from build123d import *

# Parameters (mm, degrees)
BASE_FLANGE1_DEPTH = 27
SKETCH2_R          = 3
CUT_EXTRUDE1_DEPTH = 10
CHAMFER1_SIZE      = 2


# Sheet-metal steps are written as plain solids
with BuildPart() as part:
    # Sketch1 → Base-Flange1 (new, symmetric)
    with BuildSketch(Plane.XY):
        with BuildLine():
            Line((95, -32.5), (81, -32.5))
            ThreePointArc((81, -32.5), (78.878679656, -31.621320344), (78, -29.5))
            Line((78, -29.5), (78, 31))
            ThreePointArc((78, 31), (77.560660172, 32.060660172), (76.5, 32.5))
            Line((76.5, 32.5), (-76.5, 32.5))
            ThreePointArc((-76.5, 32.5), (-77.560660172, 32.060660172), (-78, 31))
            Line((-78, 31), (-78, -29.5))
            ThreePointArc((-78, -29.5), (-78.878679656, -31.621320344), (-81, -32.5))
            Line((-81, -32.5), (-95, -32.5))
            Line((-95, -32.5), (-95, -31))
            Line((-95, -31), (-81, -31))
            ThreePointArc((-81, -31), (-79.939339828, -30.560660172), (-79.5, -29.5))
            Line((-79.5, -29.5), (-79.5, 31))
            ThreePointArc((-79.5, 31), (-78.621320344, 33.121320344), (-76.5, 34))
            Line((-76.5, 34), (76.5, 34))
            ThreePointArc((76.5, 34), (78.621320344, 33.121320344), (79.5, 31))
            Line((79.5, 31), (79.5, -29.5))
            ThreePointArc((79.5, -29.5), (79.939339828, -30.560660172), (81, -31))
            Line((81, -31), (95, -31))
            Line((95, -31), (95, -32.5))
        make_face()
    extrude(amount=BASE_FLANGE1_DEPTH, both=True)

    # Sketch2 → Cut-Extrude1 (cut)
    with BuildSketch(Plane(origin=(0, -31, 0), x_dir=(1, 0, 0), z_dir=(0, 1, 0))):
        with Locations(Location((-87.5, -15, 0), (0, 0, 270))):
            Circle(SKETCH2_R)
        with Locations(Location((87.5, -15, 0), (0, 0, 90))):
            Circle(SKETCH2_R)
        with Locations(Location((87.5, 15, 0), (0, 0, 270))):
            Circle(SKETCH2_R)
        with Locations(Location((-87.5, 15, 0), (0, 0, 90))):
            Circle(SKETCH2_R)
    extrude(amount=-CUT_EXTRUDE1_DEPTH, mode=Mode.SUBTRACT)

    # Chamfer1
    chamfer1_edges = [part.edges().sort_by_distance(p)[0] for p in [
        (95, -31.75, -27),
        (-95, -31.75, -27),
        (95, -31.75, 27),
        (-95, -31.75, 27),
    ]]
    chamfer(chamfer1_edges, length=CHAMFER1_SIZE)


solid = part.part
Input: part model. Units: mm. Frame: model coordinates. A direction names the side the tool comes from. Coordinates: 2 decimals unless noted, no trailing zeros. Order: outer loops, then holes, each group sorted by start corner. A loop starts at its lowest first (then second) coordinate and runs counter-clockwise, first axis right, second up. Notation, with made-up numbers: M 53.5,40.5 L 62.5,40.5 A22 ccw 62.5,47.5 Z; hole C 57.25,-27.5 d7. An arc over 180 degrees is marked long. Answer in a Markdown table with one row per item.
(1) Section query D-D, the plane z = 7. Output: boundary loops of the cut face in (x, y).
Numbers:
| item | result |
|---|---|
| outline | M -95,-32.5 L -81,-32.5 A3 ccw -78,-29.5 L -78,31 A1.5 cw -76.5,32.5 L 76.5,32.5 A1.5 cw 78,31 L 78,-29.5 A3 ccw 81,-32.5 L 95,-32.5 L 95,-31 L 81,-31 A1.5 cw 79.5,-29.5 L 79.5,31 A3 ccw 76.5,34 L -76.5,34 A3 ccw -79.5,31 L -79.5,-29.5 A1.5 cw -81,-31 L -95,-31 Z |
(2) Section query B-B, the plane z = -15. Output: boundary loops of the cut face in (x, y).
Numbers:
| item | result |
|---|---|
| outline | M -95,-32.5 L -90.5,-32.5 L -90.5,-31 L -95,-31 Z; M -84.5,-32.5 L -81,-32.5 A3 ccw -78,-29.5 L -78,31 A1.5 cw -76.5,32.5 L 76.5,32.5 A1.5 cw 78,31 L 78,-29.5 A3 ccw 81,-32.5 L 84.5,-32.5 L 84.5,-31 L 81,-31 A1.5 cw 79.5,-29.5 L 79.5,31 A3 ccw 76.5,34 L -76.5,34 A3 ccw -79.5,31 L -79.5,-29.5 A1.5 cw -81,-31 L -84.5,-31 Z; M 90.5,-32.5 L 95,-32.5 L 95,-31 L 90.5,-31 Z |
(3) Access query for faces 1 (the flat face through (-79.5, 0, 0)), 2 (the flat face through (88, -31, 0)), 3 (the flat face through (-78, 1, 0)). Directions: +Z, -Z, +X, -X, +Y, -Y. A direction counts if a zero-diameter tool reaches every point of the face in a straight line with its end or side. Return the directions, or none.
Numbers:
| item | result |
|---|---|
| face 1 | +Z, -Z, -X, +Y |
| face 2 | +Z, -Z, +X, +Y |
| face 3 | +Z, -Z, -Y |
(4) Section query C-C, the plane x = -87.5. Output: boundary loops of the cut face in (y, z), plus the area to 3 significant figures.
Numbers:
| item | result |
|---|---|
| outline | M -32.5,-27 L -31,-27 L -31,-18 L -32.5,-18 Z; M -32.5,-12 L -31,-12 L -31,12 L -32.5,12 Z; M -32.5,18 L -31,18 L -31,27 L -32.5,27 Z |
| area | 63.0 mm^2 |
(5) Contact query for flat-ended pins moving along their axis: pin 1 Ø6 at (y, z) = (-20.5, -4) entering from -X; pin 2 Ø16 at (y, z) = (-7.5, -5.5) entering from +X; pin 3 Ø5 at (x, z) = (87.5, 15) entering from +Y; pin 4 Ø7 at (x, z) = (90, -7) entering from +Y. Output: stop coordinate, or through.
Numbers:
| item | result |
|---|---|
| pin 1 | stops at x = -79.5 |
| pin 2 | stops at x = 79.5 |
| pin 3 | passes through |
| pin 4 | stops at y = -31 |
(6) Draft query along X for faces 4 (the flat face through (79.5, 1, 0)), 5 (the flat face through (1, 32.5, 0)), 6 (the flat face through (-88, -31, 0)). Return one class per face: pulls with the +X half, pulls with the -X half, needs draft (parallel to the pull), parting line crosses it, or undercut.
Numbers:
| item | result |
|---|---|
| face 4 | pulls with the +X half |
| face 5 | undercut |
| face 6 | needs draft |
(7) Section query A-A, the plane y = -15. Output: boundary loops of the cut face in (x, z), plus the area to 3 significant figures.
Numbers:
| item | result |
|---|---|
| outline | M -79.5,-27 L -78,-27 L -78,27 L -79.5,27 Z; M 78,-27 L 79.5,-27 L 79.5,27 L 78,27 Z |
| area | 162 mm^2 |
(8) Material intervals for line 1 (X direction, y = -1, z = -2); line 2 (X direction, y = -31.55, z = -15); line 3 (X direction, y = -31.8, z = 15), sorted ascending. Write a range as [from, to].
Numbers:
| item | result |
|---|---|
| line 1 | x = [-79.5, -78], [78, 79.5] |
| line 2 | x = [-95, -90.5], [-84.5, -78.81], [78.81, 84.5], [90.5, 95] |
| line 3 | x = [-95, -90.5], [-84.5, -79.07], [79.07, 84.5], [90.5, 95] |
